```python
from build123d import *

# Parameters (mm, degrees)
BOSS_EXTRUDE1_DEPTH = 2
BOSS_EXTRUDE2_START = -16
BOSS_EXTRUDE2_DEPTH = 2
SKETCH3_W           = 19
SKETCH3_H           = 3
BOSS_EXTRUDE3_DEPTH = 8
FILLET1_R           = 4
SKETCH5_W           = 1
SKETCH5_H           = 3
HOLE1_AT_2_COUNT    = 2
HOLE1_AT_2_PITCH    = 11
CUT_EXTRUDE1_START  = 2
SKETCH6_R           = 1
CUT_EXTRUDE1_DEPTH  = 2
FILLET2_R           = 1


# Read off the part's stored shape, not the designer's step: Boss-Extrude2
with BuildPart() as part:
    # Sketch1 → Boss-Extrude1 (new body)
    with BuildSketch(Plane.ZY.offset(14)):
        with BuildLine():
            Line((12.85, 10.15), (-1.5, 10.15))
            ThreePointArc((-1.5, 10.15), (-6.15, 5.5), (-1.5, 0.85))
            Line((-1.5, 0.85), (12.85, 0.85))
            Line((12.85, 0.85), (12.85, 0.5))
            ThreePointArc((12.85, 0.5), (17.5, -4.15), (22.15, 0.5))
            Line((22.15, 0.5), (22.15, 10.5))
            ThreePointArc((22.15, 10.5), (17.5, 15.15), (12.85, 10.5))
            Line((12.85, 10.5), (12.85, 10.15))
        make_face()
        with BuildLine():
            Line((13.85, 8.15), (-1.5, 8.15))
            ThreePointArc((-1.5, 8.15), (-4.15, 5.5), (-1.5, 2.85))
            Line((-1.5, 2.85), (13.85, 2.85))
            ThreePointArc((13.85, 2.85), (14.557106781, 2.557106781), (14.85, 1.85))
            Line((14.85, 1.85), (14.85, 0.5))
            ThreePointArc((14.85, 0.5), (17.5, -2.15), (20.15, 0.5))
            Line((20.15, 0.5), (20.15, 10.5))
            ThreePointArc((20.15, 10.5), (17.5, 13.15), (14.85, 10.5))
            Line((14.85, 10.5), (14.85, 9.15))
            ThreePointArc((14.85, 9.15), (14.557106781, 8.442893219), (13.85, 8.15))
        make_face(mode=Mode.SUBTRACT)
    extrude(amount=BOSS_EXTRUDE1_DEPTH)

    # Boss-Extrude2 outline → Boss-Extrude2 (add)
    with BuildSketch(Plane.YZ.offset(BOSS_EXTRUDE2_START)):
        with BuildLine():
            Line((-10, 12.85), (-10, -6.15))
            Line((-10, -6.15), (5.5, -6.15))
            ThreePointArc((5.5, -6.15), (2.211953467, -4.788046533), (0.85, -1.5))
            Line((0.85, -1.5), (0.85, 12.85))
            Line((0.85, 12.85), (-10, 12.85))
        make_face()
    extrude(amount=BOSS_EXTRUDE2_DEPTH)

    # Sketch3 → Boss-Extrude3 (add)
    with BuildSketch(Plane.ZY.offset(16)):
        with Locations((3.35, -8.5)):
            Rectangle(SKETCH3_W, SKETCH3_H)
    extrude(amount=BOSS_EXTRUDE3_DEPTH)

    # Fillet1
    fillet1_edges = [part.edges().sort_by_distance(p)[0] for p in [
        (-24, -8.5, 12.85),
        (-24, -8.5, -6.15),
        (-16, -7, 3.35),
    ]]
    fillet(fillet1_edges, radius=FILLET1_R - 0.0001)  # a hair under: the kernel refuses the full size

    # Sketch5 → Hole1 (revolve, cut)
    with BuildSketch(Plane(origin=(-20, -7, -2.15), x_dir=(0, 0, 1), z_dir=(1, 0, 0))):
        with Locations((0.5, 1.5)):
            Rectangle(SKETCH5_W, SKETCH5_H)
    hole1 = revolve(axis=Axis((-20, -117, -2.15), (0, 1, 0)), mode=Mode.SUBTRACT)

    # Hole1 at 2: Hole1 ×2
    with Locations(*[(0, 0, i * HOLE1_AT_2_PITCH) for i in range(1, HOLE1_AT_2_COUNT)]):
        add(hole1, mode=Mode.SUBTRACT)

    # Sketch6 → Cut-Extrude1 (cut)
    with BuildSketch(Plane(origin=(0, -7, 0), x_dir=(1, 0, 0), z_dir=(0, 1, 0)).offset(CUT_EXTRUDE1_START)):
        with Locations(Location((-20, -8.85, 0), (0, 0, 270))):
            Circle(SKETCH6_R)
        with Locations(Location((-20, 2.15, 0), (0, 0, 270))):
            Circle(SKETCH6_R)
    extrude(amount=-CUT_EXTRUDE1_DEPTH, mode=Mode.SUBTRACT)

    # Fillet2
    fillet2_edges = [part.edges().sort_by_distance(p)[0] for p in [
        (-15, 10.15, 12.85),
    ]]
    fillet(fillet2_edges, radius=FILLET2_R)
    fillet2_2_edges = [part.edges().sort_by_distance(p)[0] for p in [
        (-15, 0.5, 12.85),
    ]]
    fillet(fillet2_2_edges, radius=FILLET2_R)


solid = part.part
```
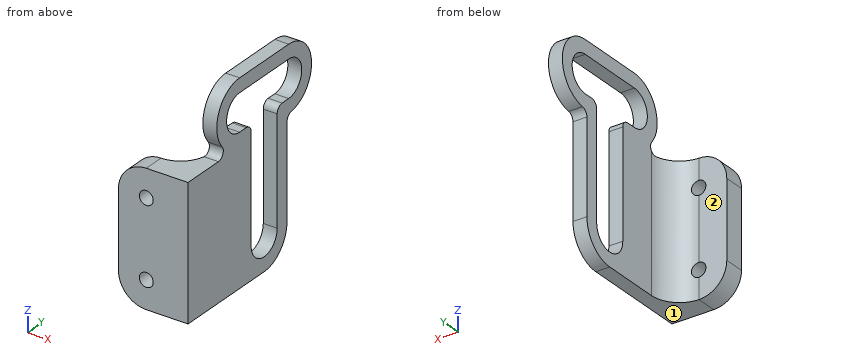
The model under review builds one solid part; all positions refer to its coordinate system, in mm. Face numbers are marked on the shaded views. A direction names the side the tool comes from. Coordinates: 2 decimals unless noted, no trailing zeros. Write each loop counter-clockwise with the first axis right and the second up, starting at its lowest first coordinate (ties: lowest second). Pieces come first, ordered by that corner, then holes.
1) We need section D-D on z = 8.5. State the section outline as (x, y) points.
2) To check wall thickness, follow probe 1 along Z at (x, y) = (-20, -8.9); probe 2 along X at (y, z) = (-7.95, -2.15); probe 3 along Y at (x, z) = (-15.5, 6). State the ranges of each line that lie inside material, in increasing order.
3) We need section A-A on z = 17.5. State the section outline as (x, y) points, then the cut area to 3 significant figures.
4) Clearance check with flat-ended pins moving along their axes: pin 1 Ø1 at (x, y) = (-15, 8) entering from -Z; pin 2 Ø9.5 at (y, z) = (1, 6) entering from -X; pin 3 Ø1.2 at (x, z) = (-21.5, 3.5) entering from +Y. State where each tip first meets the part, or that it passes through.
5) We need section B-B on y = 3.25. State the section outline as (x, z) points.
6) We need section C-C on x = -20.5. State the section outline as (y, z) points.
7) Machinability: for the marked faces 1 and 2, which of the approach directions +Z, -Z, +X, -X, +Y, -Y give a long, thin tool a straight path to every point of the face, cutting with its end or side? Answer none if there is none.
Answer list:
1. outline: (-24, -10) - (-20.94, -10) - (-20.94, -7) - (-24, -7) - close; (-19.06, -10) - (-14, -10) - (-14, 2.85) - (-16, 2.85) - (-16, -3) arc R4 cw to (-19.06, -6.89) - close; (-16, 8.15) - (-14, 8.15) - (-14, 10.15) - (-16, 10.15) - close
2. probe 1: z = -6.15 to -3.15, -1.15 to 7.85, 9.85 to 12.85
2. probe 2: x = -24 to -21, -19 to -14
2. probe 3: y = -10 to 2.85, 8.15 to 10.15
3. outline: (-16, -4.15) - (-14, -4.15) - (-14, -2.15) - (-16, -2.15) - close; (-16, 13.15) - (-14, 13.15) - (-14, 15.15) - (-16, 15.15) - close
3. area: 8.00 mm2
4. pin 1: stops at z = -5.7
4. pin 2: stops at x = -16.07
4. pin 3: stops at y = -7
5. outline: (-16, -6.15) - (-14, -6.15) - (-14, -2.9) - (-16, -2.9) - close; (-16, 20.15) - (-14, 20.15) - (-14, 22.15) - (-16, 22.15) - close
6. outline: (-10, -6.12) - (-7, -6.12) - (-7, -3.02) - (-10, -3.02) - close; (-10, -1.28) - (-7, -1.28) - (-7, 7.98) - (-10, 7.98) - close; (-10, 9.72) - (-7, 9.72) - (-7, 12.82) - (-10, 12.82) - close
7. face 1: -Z, +X, -X, +Y, -Y
7. face 2: +Z, -Z, -X, +Y
